Autodesk Inventor part; units mm, degrees
ref_plane "YZ Plane" through (0, 0, 0) normal (1, 0, 0) x (0, 1, 0)
ref_plane "XZ Plane" through (0, 0, 0) normal (0, 1, 0) x (-1, 0, 0)
ref_plane "XY Plane" through (0, 0, 0) normal (0, 0, 1) x (1, 0, 0)
sketch "Sketch1" plane through (0, 0, 0) normal (1, 0, 0) x (0, 1, 0)
  line L0 (0, 0) -> (863.6, 0)
  line L1 (863.6, 0) -> (863.6, -19.05)
  line L2 (863.6, -19.05) -> (0, -19.05)
  line L3 (0, -19.05) -> (0, 0)
  dimension "d0" = 863.6
  dimension "d1" = 19.05
extrude "Extrusion1" add sketch "Sketch1" against normal blind 38.1
sketch "Sketch2" plane through (0, 0, 0) normal (1, 0, 0) x (0, 0, -1)
  line L0 (19.05, 0) -> (0, 0)
  line L1 (19.05, 0) -> (12.7, 0)
  line L2 (12.7, 0) -> (12.7, 38.1)
  line L3 (12.7, 38.1) -> (19.05, 38.1)
  line L4 (19.05, 38.1) -> (19.05, 0)
  point P0 (12.7, 0)
  dimension "d4" = 6.35
  dimension "d5" = 38.1
extrude "Extrusion2" cut sketch "Sketch2" against normal blind 38.1
sketch "Sketch3" plane through (0, 0, 0) normal (1, 0, 0) x (0, 0, -1)
  line L0 (19.05, 38.1) -> (19.05, 863.6)
  line L1 (19.05, 863.6) -> (12.7, 863.6)
  line L2 (12.7, 863.6) -> (12.7, 825.5)
  line L3 (12.7, 825.5) -> (19.05, 825.5)
  line L4 (19.05, 825.5) -> (19.05, 863.6)
  point P0 (0, 0)
  dimension "d8" = 6.35
  dimension "d9" = 38.1
extrude "Extrusion3" cut sketch "Sketch3" against normal blind 38.1
sketch "Sketch4" plane through (0, 38.1, -19.05) normal (0, 0, -1) x (-1, 0, 0)
  line L0 (38.1, -38.1) -> (38.1, 825.5)
  line L1 (38.1, 0) -> (38.1, -38.1)
  line L2 (38.1, -38.1) -> (31.75, -38.1)
  line L3 (0, -38.1) -> (38.1, -38.1)
  line L4 (31.75, -38.1) -> (31.75, 825.5)
  line L5 (0, 825.5) -> (38.1, 825.5)
  line L6 (31.75, 825.5) -> (38.1, 825.5)
  line L7 (38.1, 787.4) -> (38.1, 0)
  line L8 (38.1, 825.5) -> (38.1, 0)
  dimension "d16" = 6.35
  dimension "d17" = 863.6
extrude "Extrusion4" cut sketch "Sketch4" against normal blind 9.525
properties part number "sidev2" material "Wood (Cherry)"
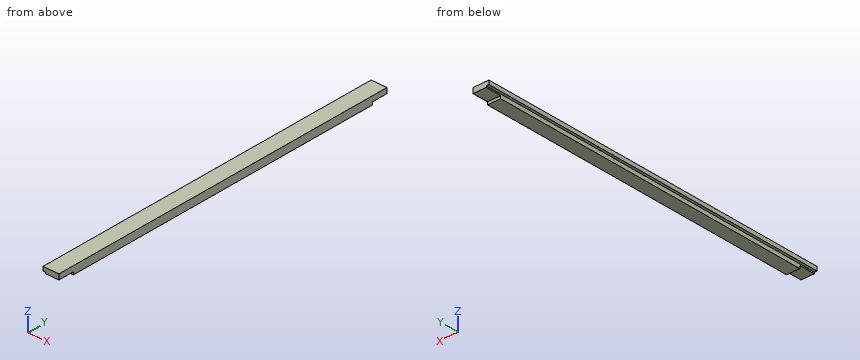
The listing builds one solid part. Answer for the finished solid, in the listing's coordinates (mm). Give positions to 0.01 mm unless a question says otherwise; leave off trailing zeros. Order: outer loops, then holes, each group sorted by start corner. A loop starts at its lowest first (then second) coordinate and runs counter-clockwise, first axis right, second up.
1) Find section A-A on x = -22.5. Write down the section's boundary in (y, z), then the cut area to 3 significant figures.
Reported:
outline: (0, -12.7) - (38.1, -12.7) - (38.1, -19.05) - (825.5, -19.05) - (825.5, -12.7) - (863.6, -12.7) - (863.6, 0) - (0, 0) - close
area: 16,000 mm2
2) Find section C-C on z = -15.75. Write down the section's boundary in (x, y), then the cut area to 3 significant figures.
Reported:
outline: (-31.75, 38.1) - (0, 38.1) - (0, 825.5) - (-31.75, 825.5) - close
area: 25,000 mm2
3) Find section B-B on y = 430. Write down the section's boundary in (x, z) (3 decimals).
Reported:
outline: (-38.1, -9.525) - (-31.75, -9.525) - (-31.75, -19.05) - (0, -19.05) - (0, 0) - (-38.1, 0) - close
4) Consider line 1 along X through (y, z) = (314, -11.5); line 2 along Y through (x, z) = (-20.5, -16.5); line 3 along Z through (x, y) = (-32, 687) (3 decimals). Determine where each line is inside the solid, lowest interval first.
Reported:
line 1: x = -31.75 to 0
line 2: y = 38.1 to 825.5
line 3: z = -9.525 to 0
5) Given P1, Ø7.5, axis at y = 251, z = -15, coming from the -X side; P2, Ø5, axis at x = -34.5, y = 261, coming from the -Z side (3 decimals); P3, Ø9.5, axis at x = -15, y = 19.5, coming from the -Z side, each flat-ended and moving along its own axis, determine where each tip first touches the part or whether it passes through.
Reported:
P1: stops at x = -31.75
P2: stops at z = -9.525
P3: stops at z = -12.7
